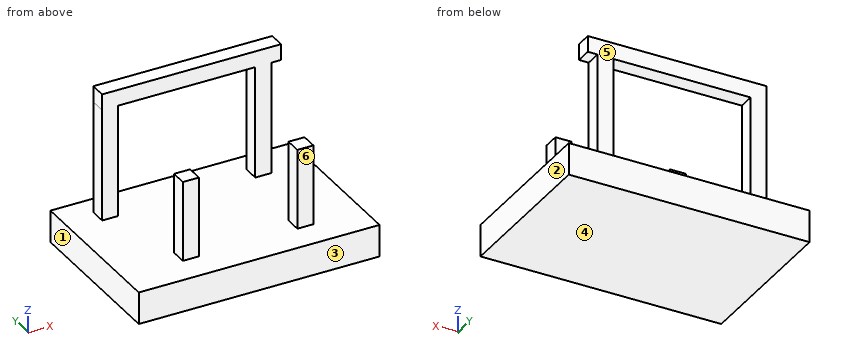
from build123d import *

# Parameters (mm, degrees)
F0_W     = 150
F0_H     = 100
F1_DEPTH = 20
F2_W     = 10
F2_H     = 10
F3_DEPTH = 70
F2_W_2   = 10.0076
F2_H_2   = 10.0076
F4_DEPTH = 50
F5_W     = 111.453053
F5_H     = 10
F6_DEPTH = 10


with BuildPart() as f1:
    # F0 (on Top) → F1 (new body)
    with BuildSketch(Plane.XY):
        with Locations((55.377272, 49.499587)):
            Rectangle(F0_W, F0_H)
    extrude(amount=F1_DEPTH)

    # F2 (on face) → F3 (join)
    with BuildSketch(Plane.XY.offset(20)):
        with Locations((5, 81.634671)):
            Rectangle(F2_W, F2_H)
        with Locations((100.377272, 81.634671)):
            Rectangle(F2_W, F2_H)
    extrude(amount=F3_DEPTH)

    # F2 (on face) → F4 (join)
    with BuildSketch(Plane.XY.offset(20)):
        with Locations((22.783541, 22.548811)):
            Rectangle(F2_W_2, F2_H_2)
        with Locations((94.102842, 22.564183)):
            Rectangle(F2_W, F2_H)
    extrude(amount=F4_DEPTH)

    # F5 (on face) → F6 (join)
    with BuildSketch(Plane.XY.offset(90)):
        with Locations((55.726526, 81.634671)):
            Rectangle(F5_W, F5_H)
    extrude(amount=F6_DEPTH)


solid = f1.part
Source: CAD feature listing. Evaluate the final solid. Frame: model axes, mm. Face numbers are marked on the shaded views. A direction names the side the tool comes from. Coordinates: 2 decimals unless noted, no trailing zeros. Loops run counter-clockwise (first coordinate to the right, second up) from the corner with the lowest first, then second, coordinate; pieces in that order, holes last. Notation, with made-up numbers: (-21.5, -4) -> (-14.5, -4) arc R32 ccw to (-14.5, 29) -> close; hole circle Ø5 at (-34.75, 84). An arc over 180 degrees is marked (long way). Answer in a Markdown table with one row per item. Add a question column.
Q1. Reachability of the marked faces 4, 5 and 6 from +Z, -Z, +X, -X, +Y, -Y: full face, straight path, thin tool, end or side. Return the list, or none.
Q2. Pull-direction query (X, two-part tool) for the marked faces 1, 2 and 3; classes: pulls with the +X half, pulls with the -X half, needs draft (parallel to the pull), parting line crosses it, or undercut.
Q3. Section A-A on z = 76.5. Return the cut outline in (x, y), and give its area (3 significant figures).
Q4. Section B-B on x = 20. Return the cut outline in (y, z).
Q5. Contact query for flat-ended pins moving along their axis: pin 1 Ø5 at (x, y) = (72, 79) entering from -Z; pin 2 Ø8 at (y, z) = (21, 48) entering from -X; pin 3 Ø5 at (y, z) = (81, 93.5) entering from -X; pin 4 Ø5 at (x, z) = (96.5, 39) entering from -Y. Output: stop coordinate, or through.
Q6. Section C-C on z = 22.5. Return the cut outline in (x, y), and give its area (3 significant figures).
Q7. Section D-D on y = 23. Return the cut outline in (x, z), and give its area (3 significant figures).
Q8. Ray query, line 1 along Y through (x, z) = (96, 57); line 2 along X through (y, z) = (82.5, 32.5); line 3 along Y through (x, z) = (24, 27.5). Return the intervals inside material, ascending.
Computed values:
| question | item | result |
|---|---|---|
| 1 | face 4 | -Z, +X, -X, +Y, -Y |
| 1 | face 5 | +Z, +X, -X, +Y |
| 1 | face 6 | +Z, +X, -X, -Y |
| 2 | face 1 | pulls with the -X half |
| 2 | face 2 | pulls with the +X half |
| 2 | face 3 | needs draft |
| 3 | outline | (0, 76.63) -> (10, 76.63) -> (10, 86.63) -> (0, 86.63) -> close; (95.38, 76.63) -> (105.38, 76.63) -> (105.38, 86.63) -> (95.38, 86.63) -> close |
| 3 | area | 200 mm^2 |
| 4 | outline | (-0.5, 0) -> (99.5, 0) -> (99.5, 20) -> (27.55, 20) -> (27.55, 70) -> (17.55, 70) -> (17.55, 20) -> (-0.5, 20) -> close; (76.63, 90) -> (86.63, 90) -> (86.63, 100) -> (76.63, 100) -> close |
| 5 | pin 1 | stops at z = 0 |
| 5 | pin 2 | stops at x = 17.78 |
| 5 | pin 3 | stops at x = 0 |
| 5 | pin 4 | stops at y = 17.56 |
| 6 | outline | (0, 76.63) -> (10, 76.63) -> (10, 86.63) -> (0, 86.63) -> close; (17.78, 17.55) -> (27.79, 17.55) -> (27.79, 27.55) -> (17.78, 27.55) -> close; (89.1, 17.56) -> (99.1, 17.56) -> (99.1, 27.56) -> (89.1, 27.56) -> close; (95.38, 76.63) -> (105.38, 76.63) -> (105.38, 86.63) -> (95.38, 86.63) -> close |
| 6 | area | 400 mm^2 |
| 7 | outline | (-19.62, 0) -> (130.38, 0) -> (130.38, 20) -> (99.1, 20) -> (99.1, 70) -> (89.1, 70) -> (89.1, 20) -> (27.79, 20) -> (27.79, 70) -> (17.78, 70) -> (17.78, 20) -> (-19.62, 20) -> close |
| 7 | area | 4,000 mm^2 |
| 8 | line 1 | y = 17.56 to 27.56, 76.63 to 86.63 |
| 8 | line 2 | x = 0 to 10, 95.38 to 105.38 |
| 8 | line 3 | y = 17.55 to 27.55 |
